```python
from build123d import *

# Parameters (mm, degrees)
BOSS_EXTRUDE1_DEPTH = 6.604
SKETCH3_W           = 6.35
SKETCH3_H           = 4.826
BOSS_EXTRUDE2_DEPTH = 6.604
CUT_EXTRUDE1_REACH  = 8.604
FILLET1_R           = 6.35


with BuildPart() as part:
    # Sketch1 → Boss-Extrude1 (new body)
    with BuildSketch(Plane.XY):
        with BuildLine():
            Line((-6.35, -5.08), (-53.975, -5.08))
            Line((-53.975, -5.08), (-53.975, -17.78))
            ThreePointArc((-53.975, -17.78), (-24.613831362, -51.146124163), (18.36841389, -62.455547599))
            ThreePointArc((18.36841389, -62.455547599), (36.58027843, -57.005297746), (49.891818948, -43.434))
            Line((49.891818948, -43.434), (39.113266772, -37.211))
            ThreePointArc((39.113266772, -37.211), (0.611966481, -44.206961223), (0, -5.08))
            Line((0, -5.08), (-6.35, -5.08))
        make_face()
    extrude(amount=BOSS_EXTRUDE1_DEPTH)

    # Sketch3 → Boss-Extrude2 (add)
    with BuildSketch(Plane.XY.offset(6.604)):
        with Locations((-47.625, -2.667)):
            Rectangle(SKETCH3_W, SKETCH3_H)
        with Locations((-28.575, -2.667)):
            Rectangle(SKETCH3_W, SKETCH3_H)
        with Locations((-9.525, -2.667)):
            Rectangle(SKETCH3_W, SKETCH3_H)
    extrude(amount=-BOSS_EXTRUDE2_DEPTH)

    # Sketch4 → Cut-Extrude1 (cut, up to next)
    with BuildSketch(Plane.XY.offset(6.604), mode=Mode.PRIVATE) as cut_extrude1_sk1:
        Polygon((-40.1828, -5.08), (-40.1828, -11.43), (-42.4688, -11.43), (-42.4688, -17.3736), (-40.1828, -17.3736), (-40.1828, -20.574), (-36.0172, -20.574), (-36.0172, -17.3736), (-33.7312, -17.3736), (-33.7312, -11.43), (-36.0172, -11.43), (-36.0172, -5.08), align=None)
    cut_extrude1_tool1 = extrude(cut_extrude1_sk1.sketch, amount=-CUT_EXTRUDE1_REACH, mode=Mode.PRIVATE) & part.part
    add(cut_extrude1_tool1.solids().sort_by_distance((-38.1, -13.293591, 6.604))[0], mode=Mode.SUBTRACT)
    # Sketch4 → Cut-Extrude1 (cut, up to next)
    with BuildSketch(Plane.XY.offset(6.604), mode=Mode.PRIVATE) as cut_extrude1_sk2:
        Polygon((-21.1328, -11.43), (-23.4188, -11.43), (-23.4188, -17.3736), (-21.1328, -17.3736), (-21.1328, -20.574), (-16.9672, -20.574), (-16.9672, -17.3736), (-14.6812, -17.3736), (-14.6812, -11.43), (-16.9672, -11.43), (-16.9672, -5.08), (-21.1328, -5.08), align=None)
    cut_extrude1_tool2 = extrude(cut_extrude1_sk2.sketch, amount=-CUT_EXTRUDE1_REACH, mode=Mode.PRIVATE) & part.part
    add(cut_extrude1_tool2.solids().sort_by_distance((-19.05, -13.293591, 6.604))[0], mode=Mode.SUBTRACT)

    # Fillet1
    fillet1_edges = [part.edges().sort_by_distance(p)[0] for p in [
        (49.891818948, -43.434, 3.302),
    ]]
    fillet(fillet1_edges, radius=FILLET1_R)


solid = part.part
```
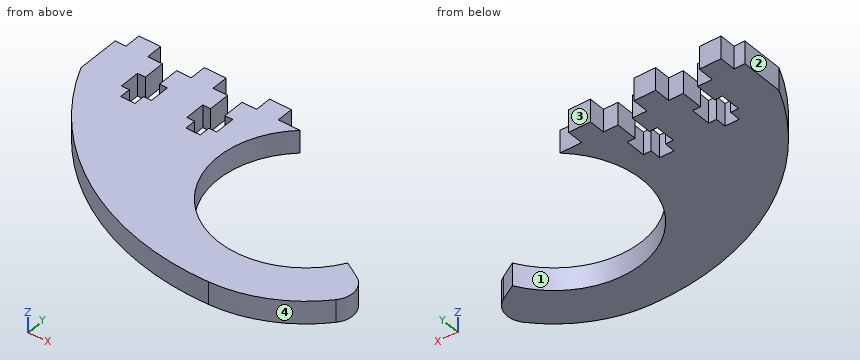
Could you check a few things on this model? Use its own coordinates, in mm. Face numbers are marked on the shaded views. Coordinates: 2 decimals unless noted, no trailing zeros. Write each loop counter-clockwise with the first axis right and the second up, starting at its lowest first coordinate (ties: lowest second). Pieces come first, ordered by that corner, then holes. Notation, with made-up numbers: (86, -11.75) -> (135, -11.75) arc R18 ccw to (135, 3.25) -> close; hole circle Ø11 at (28, 9.25). An arc over 180 degrees is marked (long way). One line per question, with ' | ' between items. Start each with the question number.
1. Will these pins go through, and if not, where does the flat tip stop? P1, Ø3, axis at x = -3.5, z = 2, coming from the +Y side; P2, Ø2.5, axis at y = -2.5, z = 4, coming from the +X side; P3, Ø0.7, axis at x = -35, z = 4, coming from the -Y side.
2. If we section it at C-C (y = -52): Please give me the cut outline in (x, z), and give its area (3 significant figures).
3. If we section it at A-A (y = -43): Please give me the cut outline in (x, z), and give its area (3 significant figures).
4. If we section it at B-B (x = 5): Please give me the cut outline in (y, z), and give its area (3 significant figures).
5. Please list where these lines run through material, in increasing order: line 1 along X through (y, z) = (-4.5, 4.25); line 2 along X through (y, z) = (-13.5, 2) (3 decimals); line 3 along Y through (x, z) = (-35, 3.5).
6. Thinking about a two-plate mould opening in X: for the marked faces 1, 2, 3 and 4, which applies, pulls with the +X half, pulls with the -X half, needs draft (parallel to the pull), parting line crosses it, or undercut?
Return value:
1) P1: stops at y = -5.08 | P2: stops at x = -6.35 | P3: stops at y = -43.75
2) outline: (-23.2, 0) -> (43.14, 0) -> (43.14, 6.6) -> (-23.2, 6.6) -> close | area: 438 mm²
3) outline: (-35.5, 0) -> (-0.76, 0) -> (-0.76, 6.6) -> (-35.5, 6.6) -> close; (34.55, 0) -> (46.53, 0) -> (46.53, 6.6) -> (34.55, 6.6) -> close | area: 309 mm²
4) outline: (-61.8, 0) -> (-47.11, 0) -> (-47.11, 6.6) -> (-61.8, 6.6) -> close | area: 97.0 mm²
5) line 1: x = -50.8 to -44.45, -31.75 to -25.4, -12.7 to -6.35 | line 2: x = -53.975 to -42.469, -33.731 to -23.419, -14.681 to -6.334 | line 3: y = -43.44 to -17.37, -11.43 to -5.08
6) face 1: undercut | face 2: pulls with the -X half | face 3: needs draft | face 4: pulls with the +X half
